Read the model definition and answer for the solid it produces. Units are mm, in the model's axes. Face numbers are marked on the shaded views. A direction names the side the tool comes from. Coordinates: 2 decimals unless noted, no trailing zeros. Order: outer loops, then holes, each group sorted by start corner. A loop starts at its lowest first (then second) coordinate and runs counter-clockwise, first axis right, second up. Notation, with made-up numbers: (-11, -22) - (4, -22) arc R22 ccw to (4, 16) - close; hole circle Ø2 at (61, 72.25). An arc over 180 degrees is marked (long way). Use one line per item in the form item = value.
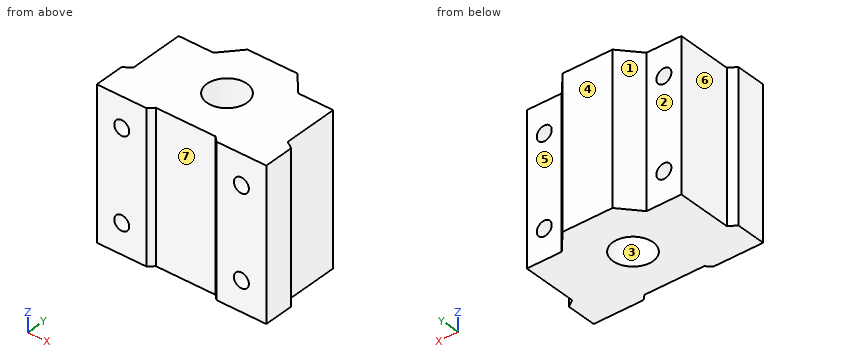
Autodesk Inventor part; units mm, degrees
ref_plane "YZ Plane" through (0, 0, 0) normal (1, 0, 0) x (0, 1, 0)
ref_plane "XZ Plane" through (0, 0, 0) normal (0, 1, 0) x (-1, 0, 0)
ref_plane "XY Plane" through (0, 0, 0) normal (0, 0, 1) x (1, 0, 0)
sketch "Sketch1" plane through (0, 0, 0) normal (0, 0, 1) x (1, 0, 0)
  circle A0 centre (0, 0) radius 4
  line L0 (-15.5, 0) -> (-15.5, 7)
  line L1 (-15.5, 7) -> (-8.5, 7)
  line L2 (-8.5, 7) -> (-5, 11)
  line L3 (-5, 11) -> (0, 11)
  line L4 (0, -4) -> (-15.5, -4) construction
  line L5 (-15.5, 0) -> (-15.5, -4)
  line L6 (-17, -11) -> (0, -11) construction
  line L7 (-17, -11) -> (-17, -5)
  line L8 (-17, -5) -> (-15.5, -4)
  line L9 (0, -4) -> (0, -11) construction
  line L10 (0, 4) -> (0, 11) construction
  line L11 (15.5, 0) -> (15.5, 7)
  line L12 (15.5, 7) -> (8.5, 7)
  line L13 (8.5, 7) -> (5, 11)
  line L14 (5, 11) -> (0, 11)
  line L15 (15.5, 0) -> (15.5, -4)
  line L16 (17, -11) -> (17, -5)
  line L17 (17, -5) -> (15.5, -4)
  line L18 (-17, -11) -> (-7, -11)
  line L19 (0, -10) -> (-6, -10)
  line L20 (-7, -11) -> (-6, -10)
  line L21 (17, -11) -> (0, -11) construction
  line L22 (0, -10) -> (6, -10)
  line L23 (7, -11) -> (6, -10)
  line L24 (7, -11) -> (17, -11)
  dimension "d0" = 8
  dimension "d1" = 15.5
  dimension "d2" = 11
  dimension "d3" = 17
  dimension "d4" = 6
  dimension "d5" = 18
  dimension "d6" = 22
  dimension "d7" = 5
  dimension "d8" = 7
  dimension "d19" = 10
  dimension "d20" = 1
  dimension "d21" = 6
extrude "Extrusion1" add sketch "Sketch1" along normal blind 30
sketch "Sketch2" plane through (-15.5, 7, 0) normal (0, 1, 0) x (1, 0, 0)
  circle A0 centre (3.5, -6) radius 1.5
  line L0 (15.5, 0) -> (15.5, -30) construction
  line L1 (32.5, 0) -> (32.5, -30) construction
  line L2 (32.5, -15) -> (-1.5, -15) construction
  line L3 (-1.5, 0) -> (-1.5, -30) construction
  line L4 (27.5, -24) -> (3.5, -24) construction
  line L5 (3.5, -24) -> (3.5, -6) construction
  line L6 (3.5, -6) -> (27.5, -6) construction
  line L7 (27.5, -6) -> (27.5, -24) construction
  line L8 (27.5, -24) -> (3.5, -6) construction
  line L9 (3.5, -24) -> (27.5, -6) construction
  circle A1 centre (27.5, -6) radius 1.5
  circle A2 centre (27.5, -24) radius 1.5
  circle A3 centre (3.5, -24) radius 1.5
  point P0 (15.5, -15)
  dimension "d11" = 3
  dimension "d12" = 24
  dimension "d13" = 18
  dimension "d14" = 3
  dimension "d15" = 3
  dimension "d16" = 3
extrude "Extrusion2" cut sketch "Sketch2" against normal through all
equation "\"d14\" = d11"
equation "\"d15\" = d11"
equation "\"d16\" = d11"
properties part number "Linear Bearing 8mm Square"
(1) Section B-B, the plane z = 6 is taken. Write down the section's boundary in (x, y), then the cut area to 3 significant figures.
Answer list:
outline = (-17, -11) - (-13.5, -11) - (-13.5, 7) - (-15.5, 7) - (-15.5, -4) - (-17, -5) - close; (-10.5, -11) - (-7, -11) - (-6, -10) - (6, -10) - (7, -11) - (10.5, -11) - (10.5, 7) - (8.5, 7) - (5, 11) - (-5, 11) - (-8.5, 7) - (-10.5, 7) - close; (13.5, -11) - (17, -11) - (17, -5) - (15.5, -4) - (15.5, 7) - (13.5, 7) - close; hole circle Ø8 at (0, 0)
area = 460 mm2
(2) Straight lines are drawn through the part: L1, parallel to Z at x = -12, y = -4.25; L2, parallel to X at y = -5.75, z = 24; L3, parallel to Y at x = 0, z = 21.25. For each, find the intervals that lie inside material, in ascending order.
Answer list:
L1 = 0 to 4.5, 7.5 to 22.5, 25.5 to 30
L2 = -17 to -13.5, -10.5 to 10.5, 13.5 to 17
L3 = -10 to -4, 4 to 11
(3) Section C-C, the plane x = 0 is taken. Write down the section's boundary in (y, z), then the cut area to 3 significant figures.
Answer list:
outline = (-10, 0) - (-4, 0) - (-4, 30) - (-10, 30) - close; (4, 0) - (11, 0) - (11, 30) - (4, 30) - close
area = 390 mm2
(4) Section D-D, the plane x = -12 is taken. Write down the section's boundary in (y, z).
Answer list:
outline = (-11, 0) - (7, 0) - (7, 4.5) - (-11, 4.5) - close; (-11, 7.5) - (7, 7.5) - (7, 22.5) - (-11, 22.5) - close; (-11, 25.5) - (7, 25.5) - (7, 30) - (-11, 30) - close
(5) Which of the six approach directions +Z, -Z, +X, -X, +Y, -Y give full straight-line access (tool end or side, diameter ignored) to the marked faces 4, 5, 6 and 7?
Answer list:
face_4 = +Z, -Z, +X, -X, +Y
face_5 = +Z, -Z, +X, +Y
face_6 = +Z, -Z, -X, +Y
face_7 = +Z, -Z, -Y
(6) Given pin 1 Ø9 at (y, z) = (3.5, 13.5) entering from +X; pin 2 Ø5 at (x, z) = (-8, 7.5) entering from +Y; pin 3 Ø10 at (x, z) = (0, 16) entering from -Y, each flat-ended and moving along its own axis, determine where each tip first touches the part or whether it passes through.
Answer list:
pin_1 = 15.5
pin_2 = 10.43
pin_3 = -10
(7) Section A-A, the plane y = 0 is taken. Write down the section's boundary in (x, z).
Answer list:
outline = (-15.5, 0) - (-4, 0) - (-4, 30) - (-15.5, 30) - close; (4, 0) - (15.5, 0) - (15.5, 30) - (4, 30) - close; hole circle Ø3 at (-12, 6); hole circle Ø3 at (-12, 24); hole circle Ø3 at (12, 6); hole circle Ø3 at (12, 24)
(8) The mould has two halves that part along X. Classify the marked faces 1, 2 and 3: +X half, -X half, draft (parallel to the pull), parting line (faces both ways), or undercut.
Answer list:
face_1 = -X half
face_2 = draft
face_3 = undercut
